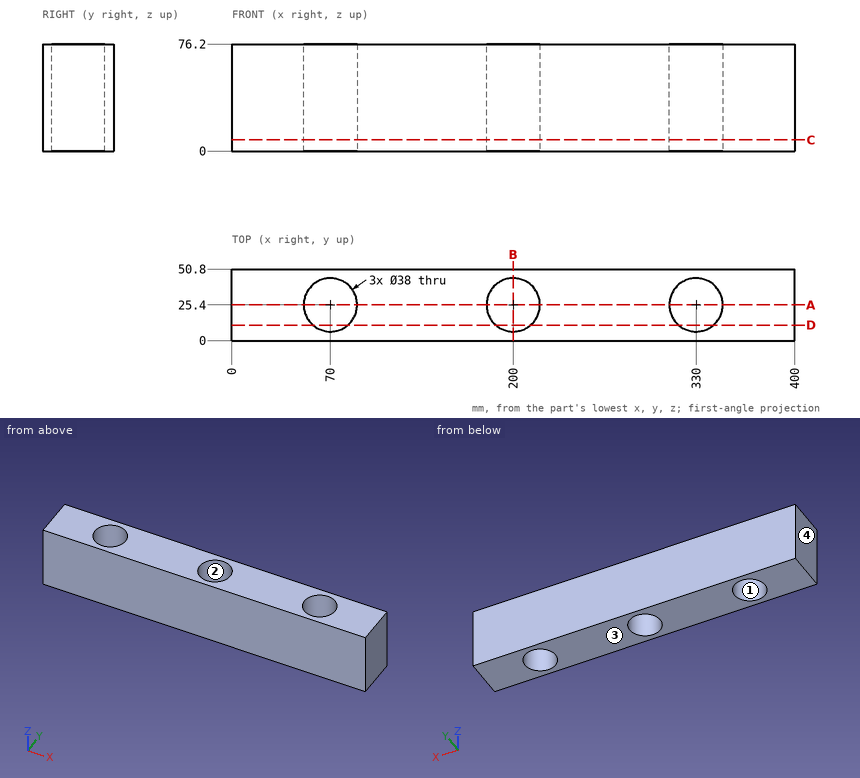
Geometry: see drawing. Coordinates: mm, zero at the bounding-box minimum. Give positions to 0.01 mm unless a question says otherwise; leave off trailing zeros. Loops run counter-clockwise (first coordinate to the right, second up) from the corner with the lowest first, then second, coordinate; pieces in that order, holes last. Notation, with made-up numbers: (-38, 58) -> (-20, 58) arc R5 ccw to (-20, 64) -> close; hole circle Ø4 at (23.5, -30.75). An arc over 180 degrees is marked (long way). Use CSV: the item, a comma, the result in double quotes.
(1) First-contact query: P1, Ø8, axis at y = 18, z = 21, coming from the -X side. Flat tip, straight axial feed; report the tip coordinate or a pass-through.
From the geometry:
P1,"x = 0"
(2) Cut plane D-D (y = 11). Output: boundary loops of the cut face in (x, z).
From the geometry:
outline,"(0, 0) -> (57.6, 0) -> (57.6, 76.2) -> (0, 76.2) -> close; (82.4, 0) -> (187.6, 0) -> (187.6, 76.2) -> (82.4, 76.2) -> close; (212.4, 0) -> (317.6, 0) -> (317.6, 76.2) -> (212.4, 76.2) -> close; (342.4, 0) -> (400, 0) -> (400, 76.2) -> (342.4, 76.2) -> close"
(3) Ray query, line 1 along X through (y, z) = (41, 29); line 2 along X through (y, z) = (18, 61); line 3 along Y through (x, z) = (330, 23). Return the intervals inside material, ascending. Write a range as [from, to].
From the geometry:
line 1,"[0, 59.15], [80.85, 189.15], [210.85, 319.15], [340.85, 400]"
line 2,"[0, 52.5], [87.5, 182.5], [217.5, 312.5], [347.5, 400]"
line 3,"[0, 6.4], [44.4, 50.8]"
(4) Cut plane C-C (z = 8). Output: boundary loops of the cut face in (x, y).
From the geometry:
outline,"(0, 0) -> (400, 0) -> (400, 50.8) -> (0, 50.8) -> close; hole circle Ø38 at (70, 25.4); hole circle Ø38 at (200, 25.4); hole circle Ø38 at (330, 25.4)"
(5) Cut plane A-A (y = 25.4). Output: boundary loops of the cut face in (x, z).
From the geometry:
outline,"(0, 0) -> (51, 0) -> (51, 76.2) -> (0, 76.2) -> close; (89, 0) -> (181, 0) -> (181, 76.2) -> (89, 76.2) -> close; (219, 0) -> (311, 0) -> (311, 76.2) -> (219, 76.2) -> close; (349, 0) -> (400, 0) -> (400, 76.2) -> (349, 76.2) -> close"
(6) Pull-direction query (X, two-part tool) for the marked faces 1, 2, 3 and 4; classes: released by +X, released by -X, zero draft, split by the parting line, or undercut.
From the geometry:
face 1,"undercut"
face 2,"undercut"
face 3,"zero draft"
face 4,"released by -X"
(7) Cut plane B-B (x = 200). Output: boundary loops of the cut face in (y, z), plus the area to 3 significant figures.
From the geometry:
outline,"(0, 0) -> (6.4, 0) -> (6.4, 76.2) -> (0, 76.2) -> close; (44.4, 0) -> (50.8, 0) -> (50.8, 76.2) -> (44.4, 76.2) -> close"
area,"975 mm^2"
